The listing builds one solid part. Answer for the finished solid, in the listing's coordinates (mm). A direction names the side the tool comes from. Coordinates: 2 decimals unless noted, no trailing zeros. Order: outer loops, then holes, each group sorted by start corner. A loop starts at its lowest first (then second) coordinate and runs counter-clockwise, first axis right, second up. Notation, with made-up numbers: (63.5, 65) -> (119.5, 65) arc R20 cw to (119.5, 70) -> close; hole circle Ø6 at (29.25, 61.25). An arc over 180 degrees is marked (long way). Write each question's results on one line, items separated by ' | '. Start each with the question number.
(1) Straight lines are drawn through the part: L1, parallel to Z at x = -2.5, y = 1; L2, parallel to Z at x = 1, y = 0.3; L3, parallel to Z at x = -6, y = 3.25. For each, find the intervals that lie inside material, in ascending order.
(2) Given pin 1 (1.1 mm diameter, centred on x = 4.5, y = 1, fed in from -Z); pin 2 (0.6 mm diameter, centred on x = -14.5, y = 1, fed in from -Z), each flat-ended and moving along its own axis, determine where each tip first touches the part or whether it passes through.
(3) The part is cut by section A-A, the plane x = 0. Give the vertices of the cut face in (y, z).
(4) A tool of negligible diameter and unlimited length cuts with its end or side. For faces 4 (the face through (-16, 0, 11)), 5 (the face through (5.5, 2, 9)), from which of +Z, -Z, +X, -X, +Y, -Y can it reach the whole face along a straight path? Write none if from no direction.
(5) The part is cut by section C-C, the plane z = -19.5. Give the vertices of the cut face in (x, y) (3 decimals), then the cut area to 3 significant figures.
(6) Determine the mould class of faces 1 (the face through (-0.59, 1.77, -13.54)), 2 (the face through (-7.064, 1.775, -25.224)), 3 (the face through (18.797, 1.825, 43.859)) for opening direction Z: +Z half, -Z half, draft (parallel to the pull), parting line (faces both ways), or undercut.
(7) The part is cut by section B-B, the plane z = 6. Give the vertices of the cut face in (x, y), then the cut area to 3 significant figures.
(8) The part is cut by section D-D, the plane z = 33. Give the vertices of the cut face in (x, y).
Autodesk Inventor part; units mm, degrees
ref_plane "YZ Plane" through (0, 0, 0) normal (1, 0, 0) x (0, 1, 0)
ref_plane "XZ Plane" through (0, 0, 0) normal (0, 1, 0) x (-1, 0, 0)
ref_plane "XY Plane" through (0, 0, 0) normal (0, 0, 1) x (1, 0, 0)
sketch "Sketch1" plane through (0, 0, 0) normal (0, 1, 0) x (-1, 0, 0)
  line L0 (20, 45) -> (-20, 45)
  line L1 (-20, 45) -> (-20, -45)
  line L2 (-20, -45) -> (20, -45)
  line L3 (20, -45) -> (20, 45)
  line L4 (20, 45) -> (-20, -45) construction
  line L5 (-20, 45) -> (20, -45) construction
  arc A0 (-20, -45) -> (20, -45) centre (0, -45) ccw
  line L6 (20, -45) -> (30, -45)
  line L7 (30, -45) -> (30, 45)
  line L8 (30, 45) -> (20, 45)
  line L9 (20, 45) -> (20, -45)
  point P0 (0, 0)
  dimension "d0" = 40
  dimension "d1" = 90
  dimension "d7" = 10
  dimension "d8" = 90
extrude "Extrusion1" add sketch "Sketch1" along normal blind 3.6
fillet "Fillet1" radius 4 3 edges at (-20, 1.8, -45) (-30, 1.8, -45) (20, 1.8, 45)
sketch "Sketch3" plane through (0, 0, 0) normal (0, -1, 0) x (1, 0, 0)
  circle A0 centre (0, -45) radius 21
  arc A1 (-19.7203, -48.3333) -> (20, -45) centre (0, -45) ccw
  point P0 (0, 0)
  dimension "d10" = 42
  dimension "d11" = 0
extrude "Extrusion3" cut sketch "Sketch3" against normal blind 10
fillet "Fillet2" radius 4 2 edges at (20, 1.8, -38.5969) (-20.9742, 1.8, -46.0397)
sketch "Sketch4" plane through (0, 0, 0) normal (0, -1, 0) x (1, 0, 0)
  circle A0 centre (-25.5, -40.5) radius 1.625
  line L0 (-24.6779, -45) -> (-26, -45)
  circle A1 centre (15.5, -19.5) radius 1.625
  circle A2 centre (15.5, 40.5) radius 1.625
  line L1 (20, 41) -> (20, -25.7906)
  arc A3 (13.44, -28.8641) -> (20, -25.7906) centre (16, -25.7906) ccw
  line L2 (-30, -41) -> (-30, 45)
  line L3 (-30, 45) -> (16, 45)
  point P0 (0, 0)
  point P1 (-30, 41)
  point P2 (-26, 45)
  dimension "d15" = 3.25
  dimension "d16" = 4.5
  dimension "d21" = 3.25
  dimension "d22" = 3.25
  dimension "d23" = 4.5
  dimension "d25" = 4.5
  dimension "d29" = 4.5
  dimension "d30" = 4.5
  dimension "d31" = 60
extrude "Extrusion4" cut sketch "Sketch4" against normal blind 7
sketch "Sketch5" plane through (0, 0, 0) normal (0, -1, 0) x (1, 0, 0)
  line L0 (-15.5, 30) -> (5.5, 30)
  line L1 (5.5, 30) -> (5.5, -13)
  line L2 (5.5, -13) -> (-15.5, -13)
  line L3 (-15.5, -13) -> (-15.5, 30)
  line L4 (-15.5, 30) -> (5.5, -13) construction
  line L5 (5.5, 30) -> (-15.5, -13) construction
  line L6 (-24.6779, -45) -> (-26, -45)
  line L7 (-30, -41) -> (-30, 45)
  point P0 (0, 0)
  point P1 (-5, 8.5)
  point P2 (-30, 41)
  dimension "d32" = 21
  dimension "d33" = 43
  dimension "d34" = 32
  dimension "d35" = 14.5
extrude "Extrusion5" cut sketch "Sketch5" against normal blind 10
sketch "Sketch6" plane through (0, 0, 0) normal (0, -1, 0) x (1, 0, 0)
  circle A0 centre (0, -18) radius 4.5
  circle A1 centre (0, 33) radius 4.5
  circle A2 centre (-10, -18) radius 4.5
  circle A3 centre (-10, 33) radius 4.5
  line L0 (5.5, 30) -> (5.5, -13)
  line L1 (5.5, -13) -> (-15.5, -13)
  point P0 (0, 0)
  dimension "d38" = 9
  dimension "d39" = 9
  dimension "d40" = 51
  dimension "d41" = 9
  dimension "d42" = 9
  dimension "d43" = 10
  dimension "d44" = 10
  dimension "d45" = 51
  dimension "d46" = 90
  dimension "d47" = 5.5
  dimension "d48" = 5
extrude "Extrusion6" cut sketch "Sketch6" against normal blind 10
fillet "Fillet3" radius 25 1 edges at (-30, 1.8, 45)
properties part number "p1"
Established:
1) L1: z = -24.15 to -21.74, -14.26 to -13, 36.74 to 45 | L2: z = -24.02 to -22.39, -13.61 to -13, 37.39 to 45 | L3: z = -24.88 to -20.06, -15.94 to -13, 30 to 30.94, 35.06 to 44.98
2) pin 1: stops at z = -24.62 | pin 2: stops at z = -30.1
3) outline: (0, -24) -> (3.6, -24) -> (3.6, -22.5) -> (0, -22.5) -> close; (0, -13.5) -> (3.6, -13.5) -> (3.6, -13) -> (0, -13) -> close; (0, 37.5) -> (3.6, 37.5) -> (3.6, 45) -> (0, 45) -> close
4) face 4: +Z, -Z, +X, -X, -Y | face 5: +Y, -Y
5) outline: (-30, 0) -> (-14.243, 0) -> (-14.243, 3.6) -> (-30, 3.6) -> close; (-5.757, 0) -> (-4.243, 0) -> (-4.243, 3.6) -> (-5.757, 3.6) -> close; (4.243, 0) -> (13.875, 0) -> (13.875, 3.6) -> (4.243, 3.6) -> close; (17.125, 0) -> (20, 0) -> (20, 3.6) -> (17.125, 3.6) -> close | area: 107 mm^2
6) face 1: undercut | face 2: -Z half | face 3: +Z half
7) outline: (-30, 0) -> (-15.5, 0) -> (-15.5, 3.6) -> (-30, 3.6) -> close; (5.5, 0) -> (20, 0) -> (20, 3.6) -> (5.5, 3.6) -> close | area: 104 mm^2
8) outline: (-26.35, 0) -> (-14.5, 0) -> (-14.5, 3.6) -> (-26.35, 3.6) -> close; (-5.5, 0) -> (-4.5, 0) -> (-4.5, 3.6) -> (-5.5, 3.6) -> close; (4.5, 0) -> (20, 0) -> (20, 3.6) -> (4.5, 3.6) -> close
